Input: part model. Units: mm. Frame: model coordinates. A direction names the side the tool comes from. Coordinates: 2 decimals unless noted, no trailing zeros. Order: outer loops, then holes, each group sorted by start corner. A loop starts at its lowest first (then second) coordinate and runs counter-clockwise, first axis right, second up. Notation, with made-up numbers: (-5, 79.5) -> (0, 79.5) arc R15 ccw to (0, 95.5) -> close; hole circle Ø1 at (49, 33). An arc over 180 degrees is marked (long way). One line per item, written item: value. Start each with the question number.
from build123d import *

# Parameters (mm, degrees)
PAD_DEPTH            = 20
BODY_PLACEMENT_ANGLE = 90


with BuildPart() as part:
    # Sketch → Pad (new body)
    with BuildSketch(Plane.XZ):
        with BuildLine():
            Line((0, 2.5), (88, 2.5))
            ThreePointArc((102.5, -12), (98.253048, -1.746952), (88, 2.5))
            Line((102.5, -12), (102.5, -22))
            Line((102.5, -22), (100, -22))
            Line((100, -22), (100, -11.5))
            ThreePointArc((100, -11.5), (96.631728, -3.368272), (88.5, 0))
            Line((88.5, 0), (0, 0))
            Line((0, 0), (0, 2.5))
        make_face()
    extrude(amount=PAD_DEPTH)


with BuildPart() as part_1:
    # Body placement: moved
    add(part.part.rotate(Axis((0, 0, 0), (-1, 0, 0)), BODY_PLACEMENT_ANGLE))


solid = part_1.part
1) Pin query (flat end, axial travel): pin 1 Ø6 at (y, z) = (-17.5, 17.5) entering from -X; pin 2 Ø2 at (y, z) = (-10.5, 3.5) entering from +X; pin 3 Ø8 at (x, z) = (23.5, 15) entering from -Y; pin 4 Ø5 at (y, z) = (-1, 14.5) entering from -X. Return the tip coordinate at first contact, or that it passes through.
2) Section query A-A, the plane z = 18. Return the cut outline in (x, y), plus the area to 3 significant figures.
3) Section query C-C, the plane y = -14.75. Return the cut outline in (x, z), plus the area to 3 significant figures.
4) Ray query, line 1 along Y through (x, z) = (5.5, 17.5); line 2 along X through (y, z) = (-20, 19); line 3 along X through (y, z) = (-2.5, 12). Return the intervals inside material, ascending. Write a range as from..to.
5) Section query B-B, the plane x = 19. Return the cut outline in (y, z).
6) Access query for faces 1 (the flat face through (100, -17, 10)), 2 (the flat face through (43, 2.5, 10)). Directions: +Z, -Z, +X, -X, +Y, -Y. A direction counts if a zero-diameter tool reaches every point of the face in a straight line with its end or side. Return the directions, or none.
Entries:
1. pin 1: stops at x = 100
1. pin 2: stops at x = 102.49
1. pin 3: stops at y = 0
1. pin 4: stops at x = 0
2. outline: (0, 0) -> (88.5, 0) arc R11.5 cw to (100, -11.5) -> (100, -22) -> (102.5, -22) -> (102.5, -12) arc R14.5 ccw to (88, 2.5) -> (0, 2.5) -> close
2. area: 295 mm2
3. outline: (100, 0) -> (102.5, 0) -> (102.5, 20) -> (100, 20) -> close
3. area: 50.0 mm2
4. line 1: y = 0..2.5
4. line 2: x = 100..102.5
4. line 3: x = 95.66..98.95
5. outline: (0, 0) -> (2.5, 0) -> (2.5, 20) -> (0, 20) -> close
6. face 1: +Z, -Z, -X, -Y
6. face 2: +Z, -Z, +X, -X, +Y
